```python
from build123d import *

# Parameters (mm, degrees)
SKETCH_1_R          = 15
SKETCH_1_R_2        = 2.1
EXTRUDE_1_DEPTH     = 3
CUT_EXTRUDE_1_DEPTH = 10


with BuildPart() as part:
    # ｽｹｯﾁ1 → ﾎﾞｽ - 押し出し1 (new body)
    with BuildSketch(Plane(origin=(0, 0, 0), x_dir=(1, 0, 0), z_dir=(0, 1, 0))):
        with Locations(Location((0, 0, 0), (0, 0, 270))):
            Circle(SKETCH_1_R)
        with Locations(Location((0, 0, 0), (0, 0, 270))):
            Circle(SKETCH_1_R_2, mode=Mode.SUBTRACT)
    extrude(amount=EXTRUDE_1_DEPTH)

    # ｽｹｯﾁ2 → ｶｯﾄ - 押し出し1 (cut)
    with BuildSketch(Plane(origin=(0, 3, 0), x_dir=(1, 0, 0), z_dir=(0, 1, 0))):
        with BuildLine():
            Line((-14.91442255, 1.6), (-6.91442255, 1.6))
            ThreePointArc((-6.91442255, 1.6), (-5.31442255, 0), (-6.91442255, -1.6))
            Line((-6.91442255, -1.6), (-14.91442255, -1.6))
            ThreePointArc((-14.91442255, -1.6), (-16.51442255, 0), (-14.91442255, 1.6))
        make_face()
    extrude(amount=-CUT_EXTRUDE_1_DEPTH, mode=Mode.SUBTRACT)


solid = part.part
```
Source: CAD feature listing. Evaluate the final solid. Frame: model axes, mm. A direction names the side the tool comes from. Coordinates: 2 decimals unless noted, no trailing zeros. Order: outer loops, then holes, each group sorted by start corner. A loop starts at its lowest first (then second) coordinate and runs counter-clockwise, first axis right, second up. Notation, with made-up numbers: M -25,-30 L 2,-30 A33 ccw 2,5 Z; hole C 26,38.25 d6. An arc over 180 degrees is marked long. Write each question's results on one line, items separated by ' | '. Start each with the question number.
1) Draft query along X for faces 1 (the face through (14.986, 1.479, 0.637)), 2 (the face through (-11, 2, 1.6)), 3 (the face through (0.631, 1.479, 2.003)). Return one class per face: released by +X, released by -X, zero draft, split by the parting line, or undercut.
2) Contact query for flat-ended pins moving along their axis: pin 1 Ø1 at (x, y) = (-6, 2) entering from -Z; pin 2 Ø1.5 at (x, y) = (-11, 2) entering from -Z. Output: stop coordinate, or through.
3) Section query B-B (x = 0). Return the cut outline in (y, z), plus the area to 3 significant figures.
4) Line query: line 1 (X direction, y = 0.85, z = 0); line 2 (Z direction, x = -9.25, y = 1); line 3 (Z direction, x = -12, y = 1.65). Output: solid intervals per line, ascending. Write a range as from..to.
5) Section query D-D (x = 3.5). Return the cut outline in (y, z).
6) Section query A-A (z = 0). Return the cut outline in (x, y).
7) Section query C-C (y = 2.15). Return the cut outline in (x, z), plus the area to 3 significant figures.
8) Access query for faces 4 (the face through (0, 0, 3)), 5 (the face through (-11, 2, -1.6)). Directions: +Z, -Z, +X, -X, +Y, -Y. A direction counts if a zero-diameter tool reaches every point of the face in a straight line with its end or side. Return the directions, or none.
Answers:
1) face 1: split by the parting line | face 2: zero draft | face 3: undercut
2) pin 1: stops at z = -13.96 | pin 2: stops at z = -10.95
3) outline: M 0,-15 L 3,-15 L 3,-2.1 L 0,-2.1 Z; M 0,2.1 L 3,2.1 L 3,15 L 0,15 Z | area: 77.4 mm^2
4) line 1: x = -5.31..-2.1, 2.1..15 | line 2: z = -11.81..-1.6, 1.6..11.81 | line 3: z = -9..-1.6, 1.6..9
5) outline: M 0,-14.59 L 3,-14.59 L 3,14.59 L 0,14.59 Z
6) outline: M -5.31,0 L -2.1,0 L -2.1,3 L -5.31,3 Z; M 2.1,0 L 15,0 L 15,3 L 2.1,3 Z
7) outline: M -14.91,-1.6 A15 ccw long -14.91,1.6 L -6.91,1.6 A1.6 cw -6.91,-1.6 Z; hole C 0,0 d4.2 | area: 663 mm^2
8) face 4: +Z, -Z, +X, -X, -Y | face 5: -X, +Y, -Y
